Could you check a few things on this drawing? It's one solid part, dimensions in mm from its lowest x, y, z. A direction names the side the tool comes from. Coordinates: 2 decimals unless noted, no trailing zeros. Loops run counter-clockwise (first coordinate to the right, second up) from the corner with the lowest first, then second, coordinate; pieces in that order, holes last.
1) Thinking about a two-plate mould opening in Y: for the marked faces 1, 2 and 3, which applies, released by +Y, released by -Y, zero draft, split by the parting line, or undercut?
2) Imagine slicing it at B-B on y = 50.5. Please give me the cut outline in (x, z) (1 decimal), plus the area to 3 significant figures.
3) For the marked faces 4, 5, 6 and 7, which set-ups out of +Z, -Z, +X, -X, +Y, -Y let a thin tool reach every point of the face, with its end or its side?
4) Imagine slicing it at C-C on z = 17.5. Please give me the cut outline in (x, y).
5) Will these pins go through, and if not, where does the flat tip stop? P1, Ø1.2, axis at y = 57, z = 41.5, coming from the +X side (1 decimal); P2, Ø20, axis at y = 25.5, z = 20, coming from the +X side; P3, Ø1.2, axis at y = 59, z = 42, coming from the -X side; P4, Ø5, axis at x = 138.81, y = 20.27, coming from the +Z side.
6) If I drill on line 1 along X through (y, z) = (63.5, 19); line 2 along Z through (x, y) = (124, 74); line 3 along Y through (x, z) = (83, 40), over which ranges is the centre line in solid material (lowest first)?
7) Imagine slicing it at A-A on z = 33.5. Please give me the cut outline in (x, y) (1 decimal).
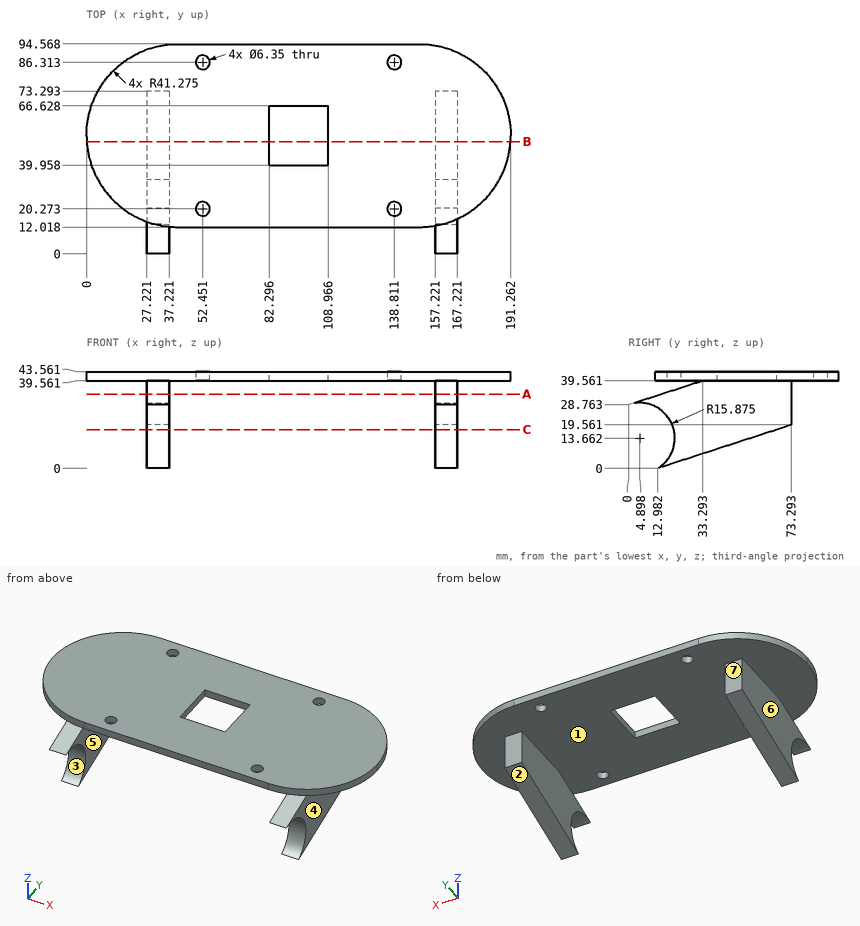
Filled in:
1. face 1: zero draft
1. face 2: released by +Y
1. face 3: undercut
2. outline: (0.1, 39.6) - (27.2, 39.6) - (27.2, 12.2) - (37.2, 12.2) - (37.2, 39.6) - (82.3, 39.6) - (82.3, 43.6) - (0.1, 43.6) - close; (109, 39.6) - (157.2, 39.6) - (157.2, 12.2) - (167.2, 12.2) - (167.2, 39.6) - (191.2, 39.6) - (191.2, 43.6) - (109, 43.6) - close
2. area: 1,210 mm2
3. face 4: -Z, +X, +Y, -Y
3. face 5: -Z, +Y, -Y
3. face 6: -Z, -X, +Y, -Y
3. face 7: -Z, +X, -X, +Y
4. outline: (27.22, 20.3) - (37.22, 20.3) - (37.22, 66.94) - (27.22, 66.94) - close; (157.22, 20.3) - (167.22, 20.3) - (167.22, 66.94) - (157.22, 66.94) - close
5. P1: stops at x = 191.1
5. P2: stops at x = 167.22
5. P3: stops at x = 0.32
5. P4: passes through
6. line 1: x = 27.22 to 37.22, 157.22 to 167.22
6. line 2: z = 39.56 to 43.56
6. line 3: y = 12.02 to 39.96, 66.63 to 94.57
7. outline: (27.2, 14.6) - (37.2, 14.6) - (37.2, 73.3) - (27.2, 73.3) - close; (157.2, 14.6) - (167.2, 14.6) - (167.2, 73.3) - (157.2, 73.3) - close
